from build123d import *

# Parameters (mm, degrees)
F1_DEPTH = 88.9
F3_DEPTH = 19.05
F5_DEPTH = 82.55


with BuildPart() as f1:
    # F0 (on Top) → F1 (new body)
    with BuildSketch(Plane.XY):
        Polygon((-87.988181, -152.4), (87.988181, -152.4), (175.976362, 0), (87.988181, 152.4), (-87.988181, 152.4), (-175.976362, 0), align=None)
    extrude(amount=F1_DEPTH)

    # F2 (on face) → F3 (cut)
    with BuildSketch(Plane(origin=(0, 0, 0), x_dir=(1, 0, 0), z_dir=(0, 0, -1))):
        Polygon((-131.982272, -76.2), (-129.782567, -74.93), (-131.687567, -71.630443), (-133.252272, -74.000295), align=None)
        Polygon((-127.877567, -78.229557), (-129.782567, -74.93), (-131.982272, -76.2), (-130.712272, -78.399705), align=None)
        Polygon((-131.687567, 71.630443), (-129.782567, 74.93), (-131.982272, 76.2), (-133.252272, 74.000295), align=None)
        Polygon((-131.982272, 76.2), (-129.782567, 74.93), (-127.877567, 78.229557), (-130.712272, 78.399705), align=None)
        Polygon((0, 149.86), (0, 152.4), (-2.54, 152.4), (-3.81, 149.86), align=None)
        Polygon((2.54, 152.4), (0, 152.4), (0, 149.86), (3.81, 149.86), align=None)
        Polygon((127.877567, 78.229557), (129.782567, 74.93), (131.982272, 76.2), (130.712272, 78.399705), align=None)
        Polygon((131.982272, 76.2), (129.782567, 74.93), (131.687567, 71.630443), (133.252272, 74.000295), align=None)
        Polygon((131.687567, -71.630443), (129.782567, -74.93), (131.982272, -76.2), (133.252272, -74.000295), align=None)
        Polygon((131.982272, -76.2), (129.782567, -74.93), (127.877567, -78.229557), (130.712272, -78.399705), align=None)
        Polygon((3.81, -149.86), (0, -149.86), (0, -152.4), (2.54, -152.4), align=None)
        Polygon((0, -152.4), (0, -149.86), (-3.81, -149.86), (-2.54, -152.4), align=None)
    extrude(amount=-F3_DEPTH, mode=Mode.SUBTRACT)

    # F4 (on face) → F5 (cut)
    with BuildSketch(Plane.XY.offset(88.9)):
        Polygon((-87.254946, -151.13), (87.254946, -151.13), (174.509892, 0), (87.254946, 151.13), (-87.254946, 151.13), (-174.509892, 0), align=None)
    extrude(amount=-F5_DEPTH, mode=Mode.SUBTRACT)


solid = f1.part
Part model, mm, in its own coordinate system. A direction names the side the tool comes from. Coordinates: 2 decimals unless noted, no trailing zeros. Loops run counter-clockwise (first coordinate to the right, second up) from the corner with the lowest first, then second, coordinate; pieces in that order, holes last. Notation, with made-up numbers: (-10, -27) -> (35, -27) arc R19 ccw to (35, 5) -> close; hole circle Ø2 at (-40, -30). An arc over 180 degrees is marked (long way). Use a Markdown table: item, result. Add a question column.
Item 1: Band-saw the part on B-B on y = 83.5. Write the cut outline in (x, z), plus the area to 3 significant figures.
Item 2: Band-saw the part on A-A on z = 70. Write the cut outline in (x, y).
Item 3: Probe probe 1 along Y at (x, z) = (-66, 23.5); probe 2 along Z at (x, y) = (-135, 50.5); probe 3 along Y at (x, z) = (126, 23.5). List the from-to ranges inside material, lowest first.
Item 4: Band-saw the part on C-C on x = 23. Write the cut outline in (y, z), plus the area to 3 significant figures.
Item 5: Pull direction Y, two halves, no side cores. Call faces 1 (the flat face through (131.366, -77.267, 43.828)), 2 (the flat face through (-131.366, 77.267, 43.828)), 3 (the flat face through (131.49, 74.51, 48.2)): +Y half, -Y half, draft (parallel to the pull), parting line (faces both ways), or undercut.
Item 6: Which spindle directions (+Z, -Z, +X, -X, +Y, -Y) get a long thin tool onto all of the face, cutting with end or side? Do faces 4 (the flat face through (1, 152.4, 44)), 5 (the flat face through (-2, 2, 6.35)). Say none if no direction does.
Item 7: Flat gauge pins, fed straight in: P1, Ø0.6, axis at x = 0, y = -152, coming from the -Z side; P2, Ø4, axis at x = 99.5, z = 66.5, coming from the -Y side; P3, Ø1, axis at y = -52.5, z = 64, coming from the -X side. Where does each tip first touch, or does it go through?
Geometry says:
| question | item | result |
|---|---|---|
| 1 | outline | (-127.77, 0) -> (127.77, 0) -> (127.77, 88.9) -> (126.3, 88.9) -> (126.3, 6.35) -> (-126.3, 6.35) -> (-126.3, 88.9) -> (-127.77, 88.9) -> close |
| 1 | area | 1,860 mm² |
| 2 | outline | (-175.98, 0) -> (-87.99, -152.4) -> (87.99, -152.4) -> (175.98, 0) -> (87.99, 152.4) -> (-87.99, 152.4) -> close; hole (-174.51, 0) -> (-87.25, -151.13) -> (87.25, -151.13) -> (174.51, 0) -> (87.25, 151.13) -> (-87.25, 151.13) -> close |
| 3 | probe 1 | -152.4 to -151.13, 151.13 to 152.4 |
| 3 | probe 2 | 0 to 6.35 |
| 3 | probe 3 | -86.56 to -84.02, 84.02 to 86.56 |
| 4 | outline | (-152.4, 0) -> (152.4, 0) -> (152.4, 88.9) -> (151.13, 88.9) -> (151.13, 6.35) -> (-151.13, 6.35) -> (-151.13, 88.9) -> (-152.4, 88.9) -> close |
| 4 | area | 2,150 mm² |
| 5 | face 1 | -Y half |
| 5 | face 2 | +Y half |
| 5 | face 3 | undercut |
| 6 | face 4 | +Z, -Z, +X, -X, +Y |
| 6 | face 5 | +Z |
| 7 | P1 | z = 19.05 |
| 7 | P2 | y = -135.93 |
| 7 | P3 | x = -145.95 |
